Design review of the part shown in the three views and the two pictorial views. Dimensions are in mm from the part's minimum x, y and z. Give positions to 0.01 mm unless a question says otherwise; leave off trailing zeros. Loops run counter-clockwise (first coordinate to the right, second up) from the corner with the lowest first, then second, coordinate; pieces in that order, holes last. Notation, with made-up numbers: M -22,54 L -17,54 A22 ccw -17,63 Z; hole C -28,0.5 d7. An arc over 180 degrees is marked long. Return JSON: item names as keys, results as strings. Group by question number.
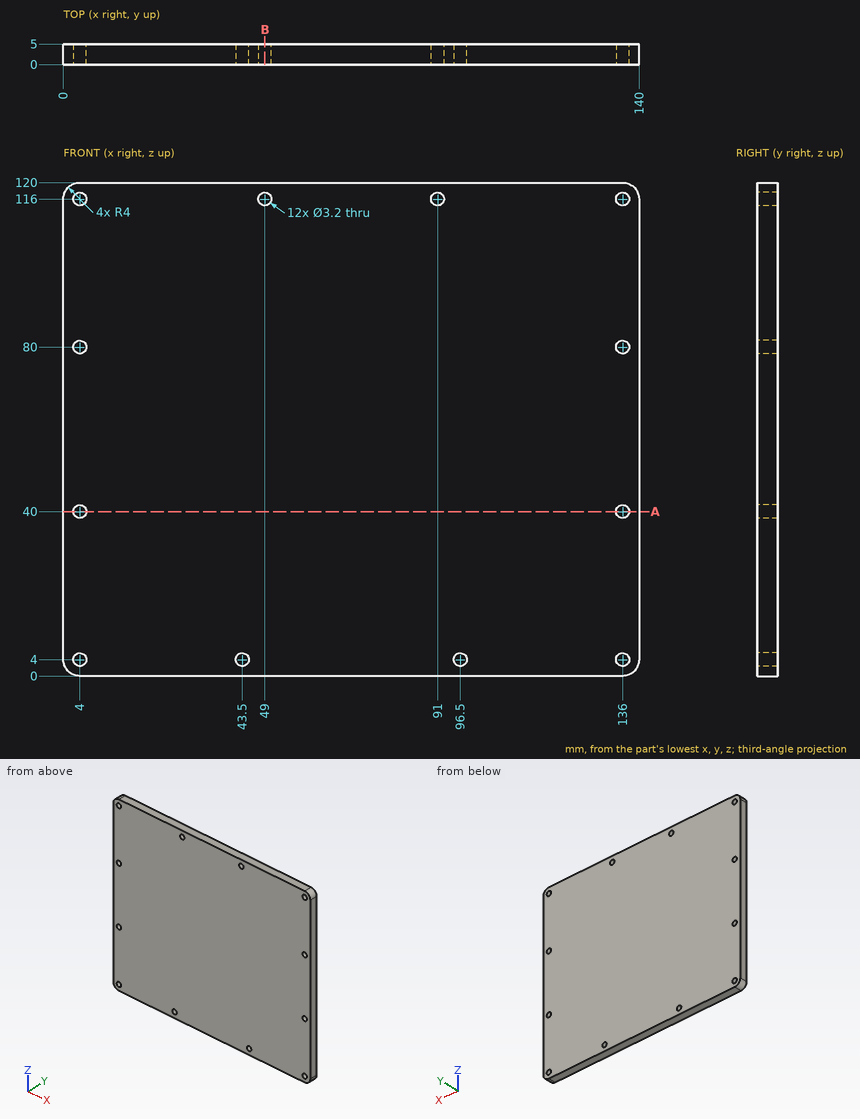
(1) Add section A-A (z = 40). Write out the cut boundary in (x, y).
(2) For pin 1 (1 mm diameter, centred on x = 27, z = 15.5, fed in from -Y); pin 2 (3 mm diameter, centred on x = 136, z = 40, fed in from +Y), all flat-tipped, find the tip position at first contact; note any pin that passes through.
(3) Add section B-B (x = 49). Write out the cut boundary in (y, z).
(4) For probe 1 along X at (y, z) = (2.15, 4); probe 2 along X at (y, z) = (1, 80); probe 3 along Z at (x, y) = (4, 1.65), list the stretches that pass through material, from the lowest coordinate up.
Verdict:
{
 "1": {"outline": "M 0,0 L 2.4,0 L 2.4,5 L 0,5 Z; M 5.6,0 L 134.4,0 L 134.4,5 L 5.6,5 Z; M 137.6,0 L 140,0 L 140,5 L 137.6,5 Z"},
 "2": {"pin 1": "stops at y = 0", "pin 2": "passes through"},
 "3": {"outline": "M 0,0 L 5,0 L 5,114.4 L 0,114.4 Z; M 0,117.6 L 5,117.6 L 5,120 L 0,120 Z"},
 "4": {"probe 1": "x = 0 to 2.4, 5.6 to 41.9, 45.1 to 94.9, 98.1 to 134.4, 137.6 to 140", "probe 2": "x = 0 to 2.4, 5.6 to 134.4, 137.6 to 140", "probe 3": "z = 0 to 2.4, 5.6 to 38.4, 41.6 to 78.4, 81.6 to 114.4, 117.6 to 120"}
}
